Design review of the part built by this model. Coordinates are the model's own, in mm. Face numbers are marked on the shaded views. A direction names the side the tool comes from. Coordinates: 2 decimals unless noted, no trailing zeros. Write each loop counter-clockwise with the first axis right and the second up, starting at its lowest first coordinate (ties: lowest second). Pieces come first, ordered by that corner, then holes. Notation, with made-up numbers: M 42,-8.75 L 62,-8.75 A20 ccw 62,21.25 Z; hole C 74,75 d1. An arc over 180 degrees is marked long. One line per question, with ' | ' between items.
from build123d import *

# Parameters (mm, degrees)
SKETCH1_R           = 10.9
BOSS_EXTRUDE1_DEPTH = 10
FILLET1_R           = 5
SKETCH2_R           = 3
CUT_EXTRUDE1_DEPTH  = 45.674489365


with BuildPart() as part:
    # Sketch1 → Boss-Extrude1 (new body)
    with BuildSketch(Plane(origin=(0, 0, 0), x_dir=(1, 0, 0), z_dir=(0, 1, 0))):
        with BuildLine():
            Line((35, 0), (-35, 0))
            Line((-35, 0), (-35, 10))
            Line((-35, 10), (-15.9, 10))
            Line((-15.9, 10), (-15.9, 20))
            ThreePointArc((-15.9, 20), (0, 35.9), (15.9, 20))
            Line((15.9, 20), (15.9, 10))
            Line((15.9, 10), (35, 10))
            Line((35, 10), (35, 0))
        make_face()
        with Locations(Location((0, 20, 0), (0, 0, 270))):
            Circle(SKETCH1_R, mode=Mode.SUBTRACT)
    extrude(amount=BOSS_EXTRUDE1_DEPTH)

    # Fillet1
    fillet1_edges = [part.edges().sort_by_distance(p)[0] for p in [
        (15.9, 5, -10),
        (-15.9, 5, -10),
    ]]
    fillet(fillet1_edges, radius=FILLET1_R)

    # Sketch2 → Cut-Extrude1 (cut, through all)
    with BuildSketch(Plane(origin=(0, 0, -10), x_dir=(-1, 0, 0), z_dir=(0, 0, -1))):
        with Locations((-30, 5)):
            Circle(SKETCH2_R)
        with Locations((30, 5)):
            Circle(SKETCH2_R)
    extrude(amount=-CUT_EXTRUDE1_DEPTH, mode=Mode.SUBTRACT)


solid = part.part
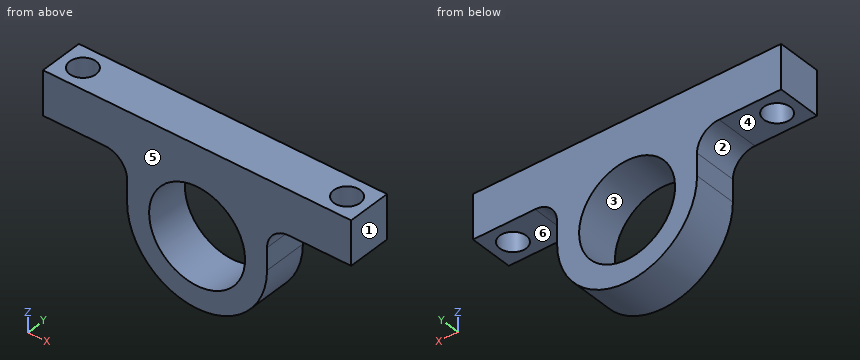
1. Take a section at B-B (x = 0). Write out the cut boundary in (y, z), then the cut area to 3 significant figures.
Answer sheet:
outline: M 0,-35.9 L 10,-35.9 L 10,-30.9 L 0,-30.9 Z; M 0,-9.1 L 10,-9.1 L 10,0 L 0,0 Z | area: 141 mm^2
2. Take a section at A-A (y = 5). Write out the cut boundary in (x, z), then the cut area to 3 significant figures.
Answer sheet:
outline: M -35,-10 L -33,-10 L -33,0 L -35,0 Z; M -27,-10 L -20.9,-10 A5 cw -15.9,-15 L -15.9,-20 A15.9 ccw 15.9,-20 L 15.9,-15 A5 cw 20.9,-10 L 27,-10 L 27,0 L -27,0 Z; M 33,-10 L 35,-10 L 35,0 L 33,0 Z; hole C 0,-20 d21.8 | area: 933 mm^2
3. To check wall thickness, follow line 1 along X through (y, z) = (8.25, -20.5); line 2 along Y through (x, z) = (-30, -2); line 3 along Z through (x, y) = (-31, 0.5). State the ranges of each line that lie inside material, in increasing order. Write a range as [from, to].
Answer sheet:
line 1: [-15.89, -10.89], [10.89, 15.89] | line 2: [0, 2], [8, 10] | line 3: [-10, 0]
4. Insertion check: pin 1 Ø5 at (y, z) = (3.5, -30.5) entering from +X; pin 2 Ø3 at (y, z) = (1.5, -26) entering from -X; pin 3 Ø2.5 at (y, z) = (6.5, -18) entering from -X. Each pin has a flat end and moves straight along its axis. Give the tip position at first contact, or say it passes through.
Answer sheet:
pin 1: x = 13.74 | pin 2: x = -15.25 | pin 3: x = -15.9
5. Take a section at C-C (z = -8). Write out the cut boundary in (x, y).
Answer sheet:
outline: M -35,0 L 35,0 L 35,10 L -35,10 Z; hole C -30,5 d6; hole C 30,5 d6
6. Take a section at D-D (x = 30). Write out the cut boundary in (y, z).
Answer sheet:
outline: M 0,-10 L 2,-10 L 2,0 L 0,0 Z; M 8,-10 L 10,-10 L 10,0 L 8,0 Z
7. Tool access review of the marked faces 4, 5 and 6: name each direction out of +Z, -Z, +X, -X, +Y, -Y from which nothing blocks a thin tool from reaching the whole face with its end or side.
Answer sheet:
face 4: -Z, -X, +Y, -Y | face 5: +Z, -Z, +X, -X, -Y | face 6: -Z, +X, +Y, -Y
8. Draft analysis for pull direction X (two halves, no side actions). For the marked faces 1, 2 and 3, state which applies: pulls with the +X half, pulls with the -X half, needs draft (parallel to the pull), parting line crosses it, or undercut.
Answer sheet:
face 1: pulls with the +X half | face 2: pulls with the -X half | face 3: undercut
